```python
from build123d import *

# Parameters (mm, degrees)
SKETCH1_R           = 7
BOSS_EXTRUDE1_DEPTH = 10
CUT_EXTRUDE1_DEPTH  = 5
BOSS_EXTRUDE2_DEPTH = 8
FILLET1_R           = 5
SKETCH4_R           = 11
CUT_EXTRUDE2_DEPTH  = 1


with BuildPart() as part:
    # Sketch1 → Boss-Extrude1 (new body)
    with BuildSketch(Plane(origin=(0, 0, 0), x_dir=(1, 0, 0), z_dir=(0, 1, 0))):
        with Locations(Location((0, 0, 0), (0, 0, 270))):
            Circle(SKETCH1_R)
    extrude(amount=BOSS_EXTRUDE1_DEPTH)

    # Sketch2 → Cut-Extrude1 (cut)
    with BuildSketch(Plane.XZ):
        Polygon((4.76388744, -2.718218128), (4.735989672, 2.76653848), (-0.027897769, 5.484756608), (-4.76388744, 2.718218128), (-4.735989672, -2.76653848), (0.027897769, -5.484756608), align=None)
    extrude(amount=-CUT_EXTRUDE1_DEPTH, mode=Mode.SUBTRACT)

    # Sketch3 → Boss-Extrude2 (add)
    with BuildSketch(Plane(origin=(0, 10, 0), x_dir=(1, 0, 0), z_dir=(0, 1, 0))):
        Polygon((20.782516215, -0.294991143), (10.646727931, 17.850691425), (-10.135788284, 18.145682568), (-20.782516215, 0.294991143), (-10.646727931, -17.850691425), (10.135788284, -18.145682568), align=None)
    extrude(amount=BOSS_EXTRUDE2_DEPTH)

    # Fillet1
    fillet1_edges = [part.edges().sort_by_distance(p)[0] for p in [
        (10.135788284, 14, 18.145682568),
        (20.782516215, 14, 0.294991143),
        (10.646727931, 14, -17.850691425),
        (-10.135788284, 14, -18.145682568),
        (-20.782516215, 14, -0.294991143),
        (-10.646727931, 14, 17.850691425),
    ]]
    fillet(fillet1_edges, radius=FILLET1_R)

    # Sketch4 → Cut-Extrude2 (cut)
    with BuildSketch(Plane(origin=(0, 18, 0), x_dir=(1, 0, 0), z_dir=(0, 1, 0))):
        with Locations(Location((0, 0, 0), (0, 0, 270))):
            Circle(SKETCH4_R)
    extrude(amount=-CUT_EXTRUDE2_DEPTH, mode=Mode.SUBTRACT)


solid = part.part
```
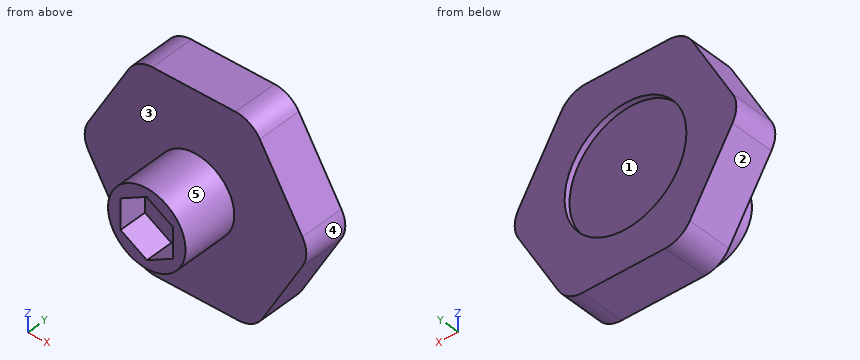
Work out the finished part from the listing and answer in its coordinate system (mm). Face numbers are marked on the shaded views. A direction names the side the tool comes from. Coordinates: 2 decimals unless noted, no trailing zeros. Loops run counter-clockwise (first coordinate to the right, second up) from the corner with the lowest first, then second, coordinate; pieces in that order, holes last.
1) Section A-A (y = 1.5) is taken. Give the vertices of the cut face in (x, z).
Results:
outline: circle Ø14 at (0, 0); hole (-4.76, 2.72) - (-4.74, -2.77) - (0.03, -5.48) - (4.76, -2.72) - (4.74, 2.77) - (-0.03, 5.48) - close
2) Section D-D (z = -9) is taken. Give the vertices of the cut face in (x, y).
Results:
outline: (-15.59, 10) - (15.59, 10) - (15.59, 18) - (6.32, 18) - (6.32, 17) - (-6.32, 17) - (-6.32, 18) - (-15.59, 18) - close
3) Flat-ended cylindrical pins translate along their axes: pin 1 (1 mm diameter, centred on x = 3, z = -3, fed in from -Y); pin 2 (4 mm diameter, centred on x = -2, y = 11.5, fed in from +Z); pin 3 (6 mm diameter, centred on x = -6.5, y = 4, fed in from -Z). Find the tip coordinate at first contact, or state that the pin passes through.
Results:
pin 1: stops at y = 5
pin 2: stops at z = 18
pin 3: stops at z = -6.06
4) Section B-B (z = 0) is taken. Give the vertices of the cut face in (x, y), plus the area to 3 significant figures.
Results:
outline: (-20.01, 10) - (-7, 10) - (-7, 0) - (-4.75, 0) - (-4.75, 5) - (4.75, 5) - (4.75, 0) - (7, 0) - (7, 10) - (20.01, 10) - (20.01, 18) - (11, 18) - (11, 17) - (-11, 17) - (-11, 18) - (-20.01, 18) - close
area: 391 mm2
5) For a pull along X with two mould halves and no side action, classify the marked faces 1, 2 and 3 as +X half, -X half, draft (parallel to the pull), parting line (faces both ways), or undercut.
Results:
face 1: undercut
face 2: -X half
face 3: draft
6) For the marked faces 4 and 5, determine the directions among +Z, -Z, +X, -X, +Y, -Y from which every point of the face is accessible in a straight line to the end or side of a thin tool.
Results:
face 4: +X, +Y, -Y
face 5: -Y
7) Section C-C (y = 10.5) is taken. Give the vertices of the cut face in (x, z).
Results:
outline: (-19.37, 2.23) arc R5 ccw to (-19.3, -2.77) - (-11.61, -15.67) arc R5 ccw to (-7.25, -18.1) - (7.76, -17.89) arc R5 ccw to (12.05, -15.33) - (19.37, -2.23) arc R5 ccw to (19.3, 2.77) - (11.61, 15.67) arc R5 ccw to (7.25, 18.1) - (-7.76, 17.89) arc R5 ccw to (-12.05, 15.33) - close
8) Consider probe 1 along X at (y, z) = (17.65, 0); probe 2 along Y at (x, z) = (5, 4); probe 3 along Y at (x, z) = (12.5, -12.5). Determine where each line is inside the solid, lowest interval first.
Results:
probe 1: x = -20.01 to -11, 11 to 20.01
probe 2: y = 0 to 17
probe 3: y = 10 to 18
